Part model, mm, in its own coordinate system. A direction names the side the tool comes from. Coordinates: 2 decimals unless noted, no trailing zeros. Write each loop counter-clockwise with the first axis right and the second up, starting at its lowest first coordinate (ties: lowest second). Pieces come first, ordered by that corner, then holes. Notation, with made-up numbers: M 15,66 L 68,66 A6 ccw 68,75 Z; hole C 51,59 d1. An arc over 180 degrees is marked long. Use a Markdown table: item, result. Add a question column.
Q1. Slice it at C-C on y = -1.25. Write the cut outline in (x, z) (3 decimals), then the cut area to 3 significant figures.
Q2. Pin check, flat tips, straight feed: pin 1 Ø1 at (y, z) = (-1, 1) entering from -X; pin 2 Ø2.5 at (x, y) = (-3.18, 11.51) entering from +Z. Stop position of each tip, or through.
Q3. Tool access for faces 1 (the flat face through (6.35, 0, 2)), 2 (the flat face through (-7, 2.921, 2)), 3 (the flat face through (0, -2.921, 2)): list every direction of +Z, -Z, +X, -X, +Y, -Y with a clear straight run to the whole face (end or side of a thin tool).
Q4. Slice it at D-D on x = 7.25. Write the cut outline in (y, z) (3 decimals).
Q5. Mould opens along Y. For faces 4 (the cylindrical face through (-3.45, 13.58, 1.57)), 5 (the flat face through (7, 2.921, 2)), 6 (the flat face through (-7.938, 7, 2)) say: released by +Y, released by -Y, zero draft, split by the parting line, or undercut.
Q6. Slice it at B-B on x = -1.5. Write the cut outline in (y, z) (3 decimals), then the cut area to 3 significant figures.
Q7. Wall check: L1, parallel to X at y = 11, z = 3.05; L2, parallel to X at y = -1, z = 2.1; L3, parallel to Y at x = -2, z = 2. Give the ranges that are in metal, low to high. Write a range as from..to.
from build123d import *

# Parameters (mm, degrees)
SKETCH1_R           = 2.0828
BOSS_EXTRUDE1_DEPTH = 3.175


with BuildPart() as part:
    # Sketch1 → Boss-Extrude1 (new body)
    with BuildSketch(Plane.XY):
        with BuildLine():
            Line((7.9375, 2.921), (0.843056521, 14.070553816))
            ThreePointArc((0.843056521, 14.070553816), (-4.506430071, 16.086474021), (-7.9375, 11.5138708))
            Line((-7.9375, 11.5138708), (-7.9375, 2.921))
            Line((-7.9375, 2.921), (-6.35, 2.921))
            Line((-6.35, 2.921), (-6.35, -2.921))
            Line((-6.35, -2.921), (6.35, -2.921))
            Line((6.35, -2.921), (6.35, 2.921))
            Line((6.35, 2.921), (7.9375, 2.921))
        make_face()
        with Locations((-3.175, 11.5138708)):
            Circle(SKETCH1_R, mode=Mode.SUBTRACT)
    extrude(amount=BOSS_EXTRUDE1_DEPTH)


solid = part.part
Recorded:
| question | item | result |
|---|---|---|
| 1 | outline | M -6.35,0 L 6.35,0 L 6.35,3.175 L -6.35,3.175 Z |
| 1 | area | 40.3 mm² |
| 2 | pin 1 | x = -6.35 |
| 2 | pin 2 | through |
| 3 | face 1 | +Z, -Z, +X, -Y |
| 3 | face 2 | +Z, -Z, -X, -Y |
| 3 | face 3 | +Z, -Z, +X, -X, -Y |
| 4 | outline | M 2.921,0 L 4.001,0 L 4.001,3.175 L 2.921,3.175 Z |
| 5 | face 4 | undercut |
| 5 | face 5 | released by -Y |
| 5 | face 6 | zero draft |
| 6 | outline | M -2.921,0 L 10.276,0 L 10.276,3.175 L -2.921,3.175 Z; M 12.752,0 L 15.972,0 L 15.972,3.175 L 12.752,3.175 Z |
| 6 | area | 52.1 mm² |
| 7 | L1 | -7.94..-5.19, -1.16..2.8 |
| 7 | L2 | -6.35..6.35 |
| 7 | L3 | -2.92..9.79, 13.23..16.13 |
